```python
from build123d import *

# Parameters (mm, degrees)
SKETCH003_W       = 92
SKETCH003_H       = 92
PAD003_DEPTH      = 26
SKETCH004_R       = 2
POCKET_DEPTH      = 26.001
POCKET_DEPTH_BACK = 0.001
FILLET_R          = 3


with BuildPart() as part:
    # Sketch003 → Pad003 (new body)
    with BuildSketch(Plane.XY):
        Rectangle(SKETCH003_W, SKETCH003_H)
    extrude(amount=PAD003_DEPTH)

    # Sketch004 (on Face5 of Pad003) → Pocket (cut, two sides)
    with BuildSketch(Plane(origin=(0, 0, 0), x_dir=(1, 0, 0), z_dir=(0, 0, -1))) as pocket_sk:
        with Locations((41.5, 41.5)):
            Circle(SKETCH004_R)
        with Locations((-41.5, 41.5)):
            Circle(SKETCH004_R)
        with Locations((41.5, -41.5)):
            Circle(SKETCH004_R)
        with Locations((-41.5, -41.5)):
            Circle(SKETCH004_R)
    extrude(amount=-POCKET_DEPTH, mode=Mode.SUBTRACT)
    extrude(pocket_sk.sketch, amount=POCKET_DEPTH_BACK, mode=Mode.SUBTRACT)

    # Fillet
    fillet_edges = [part.edges().sort_by_distance(p)[0] for p in [
        (-46, 46, 13),
        (-46, -46, 13),
        (46, -46, 13),
        (46, 46, 13),
    ]]
    fillet(fillet_edges, radius=FILLET_R)


solid = part.part
```
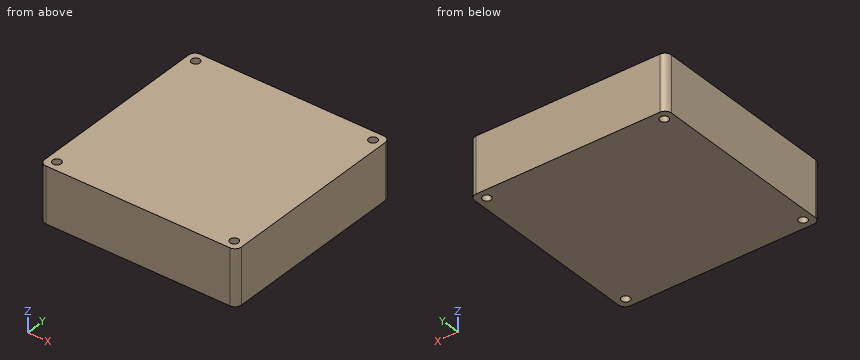
Geometry check sheet. Reference: the model listing, model coordinates, mm. Coordinates: 2 decimals unless noted, no trailing zeros. Order: outer loops, then holes, each group sorted by start corner. A loop starts at its lowest first (then second) coordinate and runs counter-clockwise, first axis right, second up.
Q1. Depth check by flat-ended pin: pin 1 Ø1.5 at (x, y) = (1, 14.5) entering from -Z. Enter the tip coordinate at first touch or a pass-through.
Reply:
pin 1: stops at z = 0
Q2. Thickness scan on probe 1 along X at (y, z) = (-41.5, 12). Record the ranges inside material, lowest first.
Reply:
probe 1: x = -46 to -43.5, -39.5 to 39.5, 43.5 to 46
Q3. Sectioned sample at A-A on x = 41.5. Record the cut outline in (y, z).
Reply:
outline: (-46, 0) - (-43.5, 0) - (-43.5, 26) - (-46, 26) - close; (-39.5, 0) - (39.5, 0) - (39.5, 26) - (-39.5, 26) - close; (43.5, 0) - (46, 0) - (46, 26) - (43.5, 26) - close
